Check sheet for the modelled part. Datum: model origin and axes. Units: mm. A direction names the side the tool comes from. Coordinates: 2 decimals unless noted, no trailing zeros. Loops run counter-clockwise (first coordinate to the right, second up) from the corner with the lowest first, then second, coordinate; pieces in that order, holes last. Notation, with made-up numbers: M 6,16 L 39,16 A20 cw 39,38 Z; hole C 83.5,17.5 d2. An arc over 180 degrees is marked long. Write each question's results on one line, items separated by ' | '. Start each with the question number.
from build123d import *

# Parameters (mm, degrees)
BOSS_EXTRUDE2_DEPTH = 21


with BuildPart() as part:
    # Sketch1 → Boss-Extrude2 (new body)
    with BuildSketch(Plane(origin=(0, 0, 0), x_dir=(1, 0, 0), z_dir=(0, 1, 0))):
        with BuildLine():
            Line((-57.106413622, -7.464824426), (-59.629413704, -7.464824426))
            ThreePointArc((-59.629413704, -7.464824426), (-60.336520485, -7.171931207), (-60.629413704, -6.464824426))
            Line((-60.629413704, -6.464824426), (-60.629413704, -6.238826501))
            ThreePointArc((-60.629413704, -6.238826501), (-60.336520485, -5.53171972), (-59.629413704, -5.238826501))
            Line((-59.629413704, -5.238826501), (-58.046413759, -5.238826501))
            Line((-58.046413759, -5.238826501), (-58.046413759, -3.741824854))
            Line((-58.046413759, -3.741824854), (-60.629413704, -3.741824854))
            ThreePointArc((-60.629413704, -3.741824854), (-62.041505931, -4.326732605), (-62.626413683, -5.738824833))
            Line((-62.626413683, -5.738824833), (-62.626413683, -6.646827448))
            ThreePointArc((-62.626413683, -6.646827448), (-62.281482952, -7.988034096), (-61.33228598, -8.996417749))
            Line((-61.33228598, -8.996417749), (-58.867053131, -10.243427026))
            ThreePointArc((-58.867053131, -10.243427026), (-58.356925281, -10.257239692), (-58.022202829, -9.87203573))
            Line((-58.022202829, -9.87203573), (-57.819413522, -9.164825189))
            Line((-57.819413522, -9.164825189), (-51.406413416, -9.164825189))
            ThreePointArc((-51.406413416, -9.164825189), (-50.913413385, -9.65782522), (-51.406413416, -10.15082525))
            Line((-51.406413416, -10.15082525), (-56.106413702, -10.15082525))
            ThreePointArc((-56.106413702, -10.15082525), (-56.813520483, -10.443718469), (-57.106413702, -11.15082525))
            Line((-57.106413702, -11.15082525), (-57.106413702, -44.164825666))
            Line((-57.106413702, -44.164825666), (-58.111413816, -44.164825666))
            Line((-58.111413816, -44.164825666), (-58.738413671, -42.164826143))
            Line((-58.738413671, -42.164826143), (-59.984413723, -42.164826143))
            Line((-59.984413723, -42.164826143), (-59.984413723, -43.864825714))
            ThreePointArc((-59.984413723, -43.864825714), (-59.398627215, -45.279039445), (-57.984413484, -45.864825952))
            Line((-57.984413484, -45.864825952), (-57.106413702, -45.864825952))
            Line((-57.106413702, -45.864825952), (-57.106413702, -50.312660842))
            ThreePointArc((-57.106413702, -50.312660842), (-56.988345829, -50.635349314), (-56.6899023, -50.805641221))
            Line((-56.6899023, -50.805641221), (-50.947861868, -51.77808339))
            ThreePointArc((-50.947861868, -51.77808339), (-50.906264859, -51.783345015), (-50.864373269, -51.785103011))
            Line((-50.864373269, -51.785103011), (-49.006412669, -51.785103011))
            ThreePointArc((-49.006412669, -51.785103011), (-48.723569957, -51.667945724), (-48.606412669, -51.385103011))
            Line((-48.606412669, -51.385103011), (-48.606412669, -50.485103011))
            ThreePointArc((-48.606412669, -50.485103011), (-48.664991313, -50.343681655), (-48.806412669, -50.285103011))
            Line((-48.806412669, -50.285103011), (-49.106412669, -50.285103011))
            Line((-49.106412669, -50.285103011), (-49.106412669, -50.685103011))
            Line((-49.106412669, -50.685103011), (-49.822333869, -50.685103011))
            ThreePointArc((-49.822333869, -50.685103011), (-49.906117049, -50.68158702), (-49.989311067, -50.671063769))
            Line((-49.989311067, -50.671063769), (-54.586309617, -49.892539951))
            ThreePointArc((-54.586309617, -49.892539951), (-54.765375734, -49.790364807), (-54.836216458, -49.596751723))
            Line((-54.836216458, -49.596751723), (-54.836216458, -48.785103011))
            ThreePointArc((-54.836216458, -48.785103011), (-54.748348492, -48.572970977), (-54.536216458, -48.485103011))
            Line((-54.536216458, -48.485103011), (-50.206412669, -48.485103011))
            ThreePointArc((-50.206412669, -48.485103011), (-49.994280635, -48.397235046), (-49.906412669, -48.185103011))
            Line((-49.906412669, -48.185103011), (-49.906412669, -16.585103011))
            Line((-49.906412669, -16.585103011), (-49.906412669, -16.185103011))
            Line((-49.906412669, -16.185103011), (-49.106412669, -16.185103011))
            Line((-49.106412669, -16.185103011), (-49.106412669, -16.585103011))
            Line((-49.106412669, -16.585103011), (-48.806412669, -16.585103011))
            ThreePointArc((-48.806412669, -16.585103011), (-48.664991313, -16.526524367), (-48.606412669, -16.385103011))
            Line((-48.606412669, -16.385103011), (-48.606412669, -15.485103011))
            ThreePointArc((-48.606412669, -15.485103011), (-48.723569957, -15.202260299), (-49.006412669, -15.085103011))
            Line((-49.006412669, -15.085103011), (-53.806412669, -15.085103011))
            Line((-53.806412669, -15.085103011), (-54.206412669, -15.085103011))
            ThreePointArc((-54.206412669, -15.085103011), (-54.489255382, -14.967945724), (-54.606412669, -14.685103011))
            Line((-54.606412669, -14.685103011), (-54.606412669, -14.585103011))
            Line((-54.606412669, -14.585103011), (-54.606412669, -12.350826013))
            ThreePointArc((-54.606412669, -12.350826013), (-54.45996606, -11.997272623), (-54.106412669, -11.850826013))
            Line((-54.106412669, -11.850826013), (-51.40641286, -11.850826013))
            ThreePointArc((-51.40641286, -11.850826013), (-49.213412067, -9.65782522), (-51.40641286, -7.464824426))
            Line((-51.40641286, -7.464824426), (-54.106412669, -7.464824426))
            Line((-54.106412669, -7.464824426), (-57.106413622, -7.464824426))
        make_face()
    extrude(amount=BOSS_EXTRUDE2_DEPTH)


solid = part.part
Item 1: Tool access check on faces 4 (the face through (-60.12, 10.35, 9.61)), 5 (the face through (-57.106, 10, 48)), 6 (the face through (-54.606, 10, 14)), 7 (the face through (-58.42, 10.35, 43.18)). Record the directions out of +Z, -Z, +X, -X, +Y, -Y that give a thin tool (end or side, any length) a straight path to the whole face; none if there is none.
Item 2: Release check for a two-part mould opening along X. For faces 1 (the face through (-62.026, 10.353, 4.311)), 2 (the face through (-52.256, 10.353, 50.287)), 3 (the face through (-60.33, 10.35, 7.18)) record: +X half, -X half, draft (parallel to the pull), parting line (faces both ways), or undercut.
Item 3: Section check B-B (z = 20). Record the cut outline in (x, y), plus the area to 3 significant figures.
Item 4: Depth check by flat-ended pin: P1, Ø1.6, axis at x = -52.5, y = 14, coming from the -Z side; P2, Ø10, axis at y = 7, z = 29.5, coming from the +X side; P3, Ø8, axis at y = 6, z = 31.5, coming from the -X side. Enter the tip coordinate at first touch or a pass-through.
Item 5: Thickness scan on line 1 (Z direction, x = -52.75, y = 13); line 2 (Z direction, x = -54, y = 16.25); line 3 (Z direction, x = -49.5, y = 7.5). Record the ranges inside material, lowest first.
Item 6: Section check A-A (x = -55.5). Record the cut outline in (y, z), plus the area to 3 significant figures.
Computed values:
1) face 4: -X, +Y, -Y | face 5: +Z, -X, +Y, -Y | face 6: +X, +Y, -Y | face 7: +Y, -Y
2) face 1: -X half | face 2: undercut | face 3: +X half
3) outline: M -57.11,0 L -49.91,0 L -49.91,21 L -57.11,21 Z | area: 151 mm²
4) P1: stops at z = 7.46 | P2: stops at x = -49.91 | P3: stops at x = -57.11
5) line 1: z = 7.46 to 9.16, 10.15 to 11.85, 15.09 to 48.49, 50.2 to 51.47 | line 2: z = 7.46 to 9.16, 10.15 to 11.85, 15.09 to 48.49, 49.99 to 51.26 | line 3: z = 8.57 to 10.74, 15.09 to 16.19, 50.69 to 51.79
6) outline: M 0,7.46 L 21,7.46 L 21,9.16 L 0,9.16 Z; M 0,10.15 L 21,10.15 L 21,51.01 L 0,51.01 Z | area: 894 mm²
